Input: part model. Units: mm. Frame: model coordinates. A direction names the side the tool comes from. Give positions to 0.01 mm unless a question says otherwise; leave off trailing zeros. Loops run counter-clockwise (first coordinate to the right, second up) from the corner with the lowest first, then second, coordinate; pieces in that order, holes last. Notation, with made-up numbers: (-12, 88.5) - (28, 88.5) arc R37 ccw to (28, 126.5) - close; hole circle Ø10 at (-35, 59.25). An arc over 180 degrees is marked (long way). Answer as a JSON object with one key per item and string values. Group by question number.
(1) Pin query (flat end, axial travel): P1, Ø10, axis at y = 34, z = -9, coming from the +X side; P2, Ø4.5, axis at x = 2, z = -3.5, coming from the +Y side; P3, Ø5, axis at x = 7, z = -5.5, coming from the +Y side. Return the tip coordinate at first contact, or that it passes through.
(2) Access query for faces 1 (the flat face through (6, 10.5, -6)), 2 (the flat face through (11.2, 5.2, 6.6)). Directions: +Z, -Z, +X, -X, +Y, -Y. A direction counts if a zero-diameter tool reaches every point of the face in a straight line with its end or side. Return the directions, or none.
(3) Material intervals for L1, parallel to Y at x = -5.5, z = 11.25; L2, parallel to X at y = 16, z = -3.75; L3, parallel to X at y = 13, z = 0, sorted ascending.
(4) Section query A-A (y = 55). Return loops of the section in (x, z), plus the area to 3 significant figures.
(5) Section query B-B (y = 69). Return loops of the section in (x, z), plus the area to 3 significant figures.
```python
from build123d import *

# Parameters (mm, degrees)
SKETCH1_R           = 7.5
BOSS_EXTRUDE1_DEPTH = 10.5
SKETCH1_3_R         = 7.5
SKETCH1_3_R_2       = 6
BOSS_EXTRUDE2_DEPTH = 67.5
SKETCH1_4_R         = 6
BOSS_EXTRUDE3_DEPTH = 82.5
SKETCH4_OUTSIDE_W   = 336.484
SKETCH4_OUTSIDE_H   = 332.462
SKETCH4_OUTSIDE_R   = 13
CUT_EXTRUDE1_DEPTH  = 82.5
CUT_EXTRUDE1_DRAFT  = -60


with BuildPart() as part:
    # Sketch1 → Boss-Extrude1 (new body)
    with BuildSketch(Plane(origin=(0, 0, 0), x_dir=(1, 0, 0), z_dir=(0, 1, 0))):
        Polygon((15.011106999, 0), (7.505553499, 13), (-7.505553499, 13), (-15.011106999, 0), (-7.505553499, -13), (7.505553499, -13), align=None)
        with Locations(Location((0, 0, 0), (0, 0, 270))):
            Circle(SKETCH1_R, mode=Mode.SUBTRACT)
    extrude(amount=BOSS_EXTRUDE1_DEPTH)

    # Sketch1<3> → Boss-Extrude2 (add)
    with BuildSketch(Plane(origin=(0, 0, 0), x_dir=(1, 0, 0), z_dir=(0, 1, 0))):
        with Locations(Location((0, 0, 0), (0, 0, 270))):
            Circle(SKETCH1_3_R)
        with Locations(Location((0, 0, 0), (0, 0, 270))):
            Circle(SKETCH1_3_R_2, mode=Mode.SUBTRACT)
    extrude(amount=BOSS_EXTRUDE2_DEPTH)

    # Sketch1<4> → Boss-Extrude3 (add)
    with BuildSketch(Plane(origin=(0, 0, 0), x_dir=(1, 0, 0), z_dir=(0, 1, 0))):
        with Locations(Location((0, 0, 0), (0, 0, 270))):
            Circle(SKETCH1_4_R)
    extrude(amount=BOSS_EXTRUDE3_DEPTH)

    # Sketch2 → Revolve1 (revolve)
    with BuildSketch(Plane.XY):
        with BuildLine():
            Line((0, 82.5), (0, 84.5))
            ThreePointArc((0, 84.5), (-3.16227766, 83.986832981), (-6, 82.5))
            Line((-6, 82.5), (0, 82.5))
        make_face()
    revolve(axis=Axis((0, 82.5, 0), (0, 1, 0)))


with BuildPart() as cut_extrude1_tool:
    # Sketch4 outside → Cut-Extrude1 (with draft: the straight prism first)
    with BuildSketch(Plane.XZ):
        Rectangle(SKETCH4_OUTSIDE_W, SKETCH4_OUTSIDE_H)
        Circle(SKETCH4_OUTSIDE_R, mode=Mode.SUBTRACT)
    extrude(amount=-CUT_EXTRUDE1_DEPTH)
    # Cut-Extrude1: the draft: its side faces are tilted about the plane it starts from
    cut_extrude1_sides = [cut_extrude1_tool.faces().sort_by_distance(p)[0] for p in [
        (0, 41.25, -166.231),
        (168.242, 41.25, 0),
        (0, 41.25, 166.231),
        (-168.242, 41.25, 0),
        (-13, 41.25, 0),
    ]]
    draft(cut_extrude1_sides, Plane.XZ, CUT_EXTRUDE1_DRAFT)


with BuildPart() as part_1:
    add(part.part)

    # Cut-Extrude1: cut by cut_extrude1_tool
    add(cut_extrude1_tool.part, mode=Mode.SUBTRACT)


solid = part_1.part
```
Recorded:
{
 "1": {"P1": "stops at x = 6.34", "P2": "stops at y = 84.34", "P3": "stops at y = 67.5"},
 "2": {"face 1": "+Y", "face 2": "+Z, +X, +Y, -Y"},
 "3": {"L1": "y = 0 to 10.5", "L2": "x = -6.5 to 6.5", "L3": "x = -7.5 to 7.5"},
 "4": {"outline": "circle Ø15 at (0, 0)", "area": "177 mm^2"},
 "5": {"outline": "circle Ø12 at (0, 0)", "area": "113 mm^2"}
}
